from build123d import *

# Parameters (mm, degrees)
F0_R     = 120
F0_R_2   = 50
F1_DEPTH = 350
F2_R     = 5


with BuildPart() as f1:
    # F0 (on Front) → F1 (new body, symmetric)
    with BuildSketch(Plane.XZ):
        with BuildLine():
            Line((-375, -400), (375, -400))
            ThreePointArc((375, -400), (427.720779, -272.720779), (555, -220))
            Line((555, -220), (1025, -220))
            ThreePointArc((1025, -220), (1245, 0), (1025, 220))
            Line((1025, 220), (555, 220))
            ThreePointArc((555, 220), (427.720779, 272.720779), (375, 400))
            Line((375, 400), (-375, 400))
            ThreePointArc((-375, 400), (-775, 0), (-375, -400))
        make_face()
        with Locations((-375, 0)):
            Circle(F0_R, mode=Mode.SUBTRACT)
        with Locations((175, 0)):
            Circle(F0_R_2, mode=Mode.SUBTRACT)
        with Locations((1025, 0)):
            Circle(F0_R, mode=Mode.SUBTRACT)
    extrude(amount=F1_DEPTH, both=True)

    # F2
    f2_edges = [f1.edges().sort_by_distance(p)[0] for p in [
        (-775, -350, 0),
        (0, -350, 400),
        (427.720779, -350, 272.720779),
        (790, -350, 220),
        (1245, -350, 0),
        (790, -350, -220),
        (427.720779, -350, -272.720779),
        (0, -350, -400),
        (-775, 350, 0),
        (0, 350, 400),
        (427.720779, 350, 272.720779),
        (790, 350, 220),
        (1245, 350, 0),
        (375, 0, -400),
        (790, 350, -220),
        (427.720779, 350, -272.720779),
        (0, 350, -400),
    ]]
    fillet(f2_edges, radius=F2_R)


solid = f1.part
Source: CAD feature listing. Evaluate the final solid. Frame: model axes, mm. A direction names the side the tool comes from. Give positions to 0.01 mm unless a question says otherwise; leave off trailing zeros. Write each loop counter-clockwise with the first axis right and the second up, starting at its lowest first coordinate (ties: lowest second). Pieces come first, ordered by that corner, then holes. Notation, with made-up numbers: M -2,71 L 49,71 A14 ccw 49,79 Z; hole C 88,35 d9. An arc over 180 degrees is marked long. Answer as a JSON object with one key per item and string values.
Q1. Cut plane B-B, the plane y = 148. Return the cut outline in (x, z), then the cut area to 3 significant figures.
Geometry check:
{"outline": "M -375,-400 L 370.07,-400 A5 ccw 375.07,-395.14 A180 cw 555,-220 L 1025,-220 A220 ccw 1025,220 L 555,220 A180 cw 375,400 L -375,400 A400 ccw Z; hole C -375,0 d240; hole C 175,0 d100; hole C 1025,0 d240", "area": "1,130,000 mm^2"}
Q2. Cut plane C-C, the plane z = 0. Count the separate pieces of the cut face and the enclosed holes in it, then the cut area to 3 significant figures.
Geometry check:
{"separate pieces": "4", "enclosed holes": "0", "area": "1,010,000 mm^2"}
Q3. Contact query for flat-ended pins moving along their axis: P1, Ø5, axis at y = 63.5, z = -68.5, coming from the -X side; P2, Ø5, axis at x = -479.5, y = 85.5, coming from the -Z side. Output: stop coordinate, or through.
Geometry check:
{"P1": "stops at x = -769.52", "P2": "stops at z = -386.78"}
Q4. Ray query, line 1 along Z through (x, y) = (175, 72); line 2 along Z through (x, y) = (1025, -9); line 3 along X through (y, z) = (205, -78). Return the intervals inside material, ascending.
Geometry check:
{"line 1": "z = -400 to -50, 50 to 400", "line 2": "z = -220 to -120, 120 to 220", "line 3": "x = -767.32 to -466.19, -283.81 to 933.81, 1116.19 to 1230.71"}
Q5. Access query for faces 5 (the face through (793, -5, 220)), 6 (the face through (905.116, 4.9, 5.276)). Directions: +Z, -Z, +X, -X, +Y, -Y. A direction counts if a zero-diameter tool reaches every point of the face in a straight line with its end or side. Return the directions, or none.
Geometry check:
{"face 5": "+Z, +X, +Y, -Y", "face 6": "+Y, -Y"}
Q6. Mould query, pull axis Z, two halves, no side actions, for faces 1 (the face through (-774.903, -4.83, 8.796)), 2 (the face through (221, 350, -82)), 3 (the face through (125.05, 4.9, 2.2)), 4 (the face through (787, -5, -220)). Classes: +Z half, -Z half, draft (parallel to the pull), parting line (faces both ways), or undercut.
Geometry check:
{"face 1": "parting line", "face 2": "draft", "face 3": "undercut", "face 4": "-Z half"}
Q7. Cut plane A-A, the plane x = 175. Return the cut outline in (y, z).
Geometry check:
{"outline": "M -350,-395 A5 ccw -345,-400 L 345,-400 A5 ccw 350,-395 L 350,-50 L -350,-50 Z; M -350,50 L 350,50 L 350,395 A5 ccw 345,400 L -345,400 A5 ccw -350,395 Z"}
